Autodesk Inventor part; units mm, degrees
ref_plane "YZ Plane" through (0, 0, 0) normal (1, 0, 0) x (0, 1, 0)
ref_plane "XZ Plane" through (0, 0, 0) normal (0, 1, 0) x (-1, 0, 0)
ref_plane "XY Plane" through (0, 0, 0) normal (0, 0, 1) x (1, 0, 0)
sketch "스케치1" plane through (0, 0, 0) normal (0, 1, 0) x (-1, 0, 0)
  circle A0 centre (0, 0) radius 23.75
  circle A1 centre (0, -23.75) radius 2.4
  line L0 (0, 0) -> (0, -23.75)
  line L1 (0, 0) -> (20.5681, 11.875)
  line L2 (0, 0) -> (23.75, 0) construction
  line L3 (0, 0) -> (-20.5681, 11.875)
  line L4 (0, 0) -> (23.75, 0) construction
  circle A2 centre (20.5681, 11.875) radius 2.4
  circle A3 centre (-20.5681, 11.875) radius 2.4
  circle A4 centre (20.5681, 11.875) radius 5
  circle A5 centre (-20.5681, 11.875) radius 5
  circle A6 centre (0, -23.75) radius 5
  circle A7 centre (0, 0) radius 12
  arc A8 (-17.6262, 15.9179) -> (17.6262, 15.9179) centre (0, 73.2705) ccw
  arc A9 (22.5984, 7.3058) -> (4.9722, -23.2237) centre (63.4541, -36.6352) ccw
  arc A10 (-4.9722, -23.2237) -> (-22.5984, 7.3058) centre (-63.4541, -36.6352) ccw
  point P0 (-4.9722, -23.2237)
  dimension "d0" = 47.5
  dimension "d8" = 10
  dimension "d1" = 4.8
  dimension "d2" = 30
  dimension "d3" = 150
  dimension "d4" = 4.8
  dimension "d5" = 4.8
  dimension "d6" = 10
  dimension "d7" = 10
  dimension "d9" = 24
  dimension "d10" = 60
  dimension "d11" = 60
  dimension "d12" = 60
sketch "스케치2" plane through (0, 0, 0) normal (0, 1, 0) x (-1, 0, 0)
  point P0 (0, 0)
extrude "돌출3" add sketch "스케치1" against normal blind 5 contours A4 L1 A2 A0 | A0 A2 A4 | A9 A6 L0 A7 L1 A4 | A6 A0 A1 | A0 A1 L0 A6 | A2 L1 A0 | A0 A2 | A4 A0 A2 L1 | L1 A7 L3 A5 A8 A4 | A1 A0 | A0 L0 A1 | A6 A10 A5 L3 A7 L0 | L0 A1 A0 A6 | L1 A2 A0 | A7 L0 L1 | L1 L3 A7 | A0 A1 L0 | A7 L3 L0 | A5 L3 A3 A0 | A0 A3 A5 | A0 A3 L3 A5 | A3 L3 A0 | A0 A3 | A0 L3 A3
sketch "스케치3" plane through (0, -5, 0) normal (0, -1, 0) x (1, 0, 0)
  point P0 (0, 0)
extrude "돌출4" add sketch "스케치1" against normal blind 10 contours A4 L1 A2 A0 | A0 A2 A4 | A9 A6 L0 A7 L1 A4 | A6 A0 A1 | A0 A1 L0 A6 | A2 L1 A0 | A0 A2 | A4 A0 A2 L1 | L1 A7 L3 A5 A8 A4 | A1 A0 | A0 L0 A1 | A6 A10 A5 L3 A7 L0 | L0 A1 A0 A6 | L1 A2 A0 | A7 L0 L1 | L1 L3 A7 | A0 A1 L0 | A7 L3 L0 | A5 L3 A3 A0 | A0 A3 A5 | A0 A3 L3 A5 | A3 L3 A0 | A0 A3 | A0 L3 A3
extrude "돌출5" add sketch "스케치1" along normal blind 55 contours A2 L1 A0 | A0 A2 | A1 A0 | A0 L0 A1 | L1 A2 A0 | A0 A1 L0 | A3 L3 A0 | A0 A3 | A0 L3 A3
sketch "스케치4" plane through (0, -10, 0) normal (0, -1, 0) x (1, 0, 0)
  circle A0 centre (0, 0) radius 8
  circle A1 centre (0, 0) radius 8
  point P0 (8, 0)
  point P1 (0, -8)
  point P2 (0, 8)
  point P3 (-8, 0)
  point P4 (-8, 0)
  point P5 (-8, 0)
  point P6 (0, 8)
  point P7 (8, 0)
  point P8 (0, -8)
  dimension "d24" = 16
  dimension "d26" = 16
sketch "스케치5" plane through (0, 0, 0) normal (0, 1, 0) x (1, 0, 0)
  circle A0 centre (0, 0) radius 8
  point P0 (8, 0)
  point P1 (0, -8)
  point P2 (-8, 0)
  point P3 (0, 8)
  dimension "d27" = 16
hole "구멍1" at (0, 0, 8) at (-8, 0, 0) at (0, 0, -8) at (8, 0, 0) direction (0, -1, 0) diameter 2.2 end through all counterbore diameter 4.2 counterbore depth 7
sketch "스케치6" plane through (0, 0, 0) normal (0, 1, 0) x (1, 0, 0)
  point P0 (0, 0)
sketch "스케치7" plane through (0, 0, 0) normal (0, 1, 0) x (1, 0, 0)
  circle A0 centre (0, 0) radius 8.95
  circle A1 centre (0, 0) radius 8
  circle A2 centre (0, 8) radius 2.1
  circle A3 centre (-8, 0) radius 2.1
  circle A4 centre (0, -8) radius 2.1
  circle A5 centre (8, 0) radius 2.1
  point P0 (8.7308, 1.9687)
  point P1 (1.9687, 8.7308)
  point P2 (-1.9687, 8.7308)
  point P3 (-8.7308, 1.9687)
  point P4 (-8.7308, -1.9687)
  point P5 (-1.9687, -8.7308)
  point P6 (1.9687, -8.7308)
  point P7 (8.7308, -1.9687)
  dimension "d37" = 16
  dimension "d36" = 17.9
  dimension "d38" = 4.2
  dimension "d41" = 360
extrude "돌출6" add sketch "스케치7" along normal blind 30 contours A5 A1 A2 A0 | A0 A4 A1 A5 | A5 A1 A4 A3 A2 | A2 A1 A3 A0 | A0 A3 A1 A4
equation "\"d19\" = d7"
equation "\"TransitionRadius\" = BendRadius"
properties part number "wheel_connection.0001"
The listing builds one solid part. Answer for the finished solid, in the listing's coordinates (mm). A direction names the side the tool comes from. Coordinates: 2 decimals unless noted, no trailing zeros. Write each loop counter-clockwise with the first axis right and the second up, starting at its lowest first coordinate (ties: lowest second). Pieces come first, ordered by that corner, then holes.
Q1. Section A-A, the plane x = 0 is taken. Write down the section's boundary in (y, z).
Returned:
outline: (-10, -28.75) - (0, -28.75) - (0, -26.15) - (55, -26.15) - (55, -21.35) - (0, -21.35) - (0, -10.1) - (-7, -10.1) - (-7, -9.1) - (-10, -9.1) - close; (-10, -6.9) - (-7, -6.9) - (-7, -5.9) - (30, -5.9) - (30, 5.9) - (-7, 5.9) - (-7, 6.9) - (-10, 6.9) - close; (-10, 9.1) - (-7, 9.1) - (-7, 10.1) - (0, 10.1) - (0, 13.27) - (-10, 13.27) - close
Q2. Given P1, Ø1.5, axis at x = 8.5, y = 28.5, coming from the +Z side; P2, Ø1.3, axis at x = -7.5, z = 0, coming from the +Y side; P3, Ø5, axis at x = 2.5, z = 1.5, coming from the +Y side, each flat-ended and moving along its own axis, determine where each tip first touches the part or whether it passes through.
Returned:
P1: stops at z = 4.48
P2: stops at y = -7
P3: stops at y = 30
Q3. Find the intervals of material crossed by line 1 along Z through (x, y) = (0, 2); line 2 along X through (y, z) = (9, 0); line 3 along Z through (x, y) = (6.5, 23), in increasing order.
Returned:
line 1: z = -26.15 to -21.35, -5.9 to 5.9
line 2: x = -5.9 to 5.9
line 3: z = -6.15 to -1.47, 1.47 to 6.15
Q4. The mould has two halves that part along X. Classify faces 5 (the cylindrical face through (9.074, -8.521, -0.238)), 6 (the cylindrical face through (11.37, -4.93, -6.85)), 7 (the flat face through (-21, 55, 12)): released by +X, released by -X, zero draft, split by the parting line, or undercut.
Returned:
face 5: undercut
face 6: released by +X
face 7: zero draft
Q5. Which of the six approach directions +Z, -Z, +X, -X, +Y, -Y give full straight-line access (tool end or side, diameter ignored) to faces 1 (the cylindrical face through (6.378, 14.79, 6.278)), 2 (the flat face through (0, 30, 0)), 3 (the cylindrical face through (22.337, 27.115, 10.253)), 4 (the cylindrical face through (-6.278, 14.79, 6.378))?
Returned:
face 1: +Z, +X, +Y
face 2: +Z, +X, -X, +Y
face 3: +Y
face 4: +Z, -X, +Y
Q6. Section B-B, the plane y = 10 is taken. Write down the section's boundary in (x, z) (3 decimals).
Returned:
outline: circle Ø4.8 at (-20.568, 11.875); (-8.731, -1.969) arc R8.95 ccw to (-1.969, -8.731) arc R2.1 cw (long way) to (1.969, -8.731) arc R8.95 ccw to (8.731, -1.969) arc R2.1 cw (long way) to (8.731, 1.969) arc R8.95 ccw to (1.969, 8.731) arc R2.1 cw (long way) to (-1.969, 8.731) arc R8.95 ccw to (-8.731, 1.969) arc R2.1 cw (long way) to start; circle Ø4.8 at (0, -23.75); circle Ø4.8 at (20.568, 11.875)
Q7. Section D-D, the plane x = 12 is taken. Write down the section's boundary in (y, z), then the cut area to 3 significant figures.
Returned:
outline: (-10, -5.77) - (0, -5.77) - (0, 14.48) - (-10, 14.48) - close
area: 203 mm2
Q8. Section C-C, the plane z = 0 is taken. Write down the section's boundary in (x, y).
Returned:
outline: (-15.94, -10) - (-9.1, -10) - (-9.1, -7) - (-10.1, -7) - (-10.1, 0) - (-15.94, 0) - close; (-6.9, -10) - (6.9, -10) - (6.9, -7) - (5.9, -7) - (5.9, 30) - (-5.9, 30) - (-5.9, -7) - (-6.9, -7) - close; (9.1, -10) - (15.94, -10) - (15.94, 0) - (10.1, 0) - (10.1, -7) - (9.1, -7) - close
